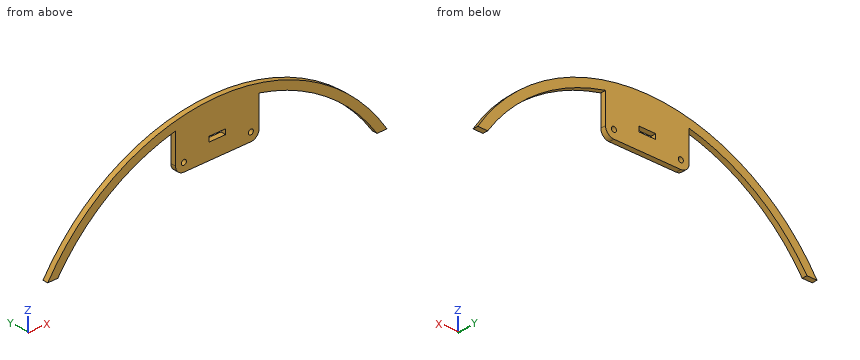
```python
from build123d import *

# Parameters (mm, degrees)
SKETCH_1_R      = 1.5
SKETCH_1_W      = 10
SKETCH_1_H      = 3
EXTRUDE_2_DEPTH = 3.125


with BuildPart() as part:
    # 草图1 → 凸台-拉伸2 (new body)
    with BuildSketch(Plane(origin=(0, 0, 0), x_dir=(1, 0, 0), z_dir=(0, 1, 0))):
        with BuildLine():
            Line((-101.350743825, 30), (-95.378054467, 30))
            ThreePointArc((-95.378054467, 30), (-64.797523096, -0.757020266), (-25, -18))
            Line((-25, -18), (-25, 0))
            ThreePointArc((-25, 0), (-23.535533906, 3.535533906), (-20, 5))
            Line((-20, 5), (20, 5))
            ThreePointArc((20, 5), (23.535533906, 3.535533906), (25, 0))
            Line((25, 0), (25, -18))
            ThreePointArc((25, -18), (64.797523096, -0.757020266), (95.378054467, 30))
            Line((95.378054467, 30), (101.350743825, 30))
            ThreePointArc((101.350743825, 30), (0, -25.750278397), (-101.350743825, 30))
        make_face()
        with Locations((-20, 0)):
            Circle(SKETCH_1_R, mode=Mode.SUBTRACT)
        with Locations((20, 0)):
            Circle(SKETCH_1_R, mode=Mode.SUBTRACT)
        with Locations((0, -6)):
            Rectangle(SKETCH_1_W, SKETCH_1_H, mode=Mode.SUBTRACT)
    extrude(amount=EXTRUDE_2_DEPTH)


solid = part.part
```
CAD build for the part. Positions are in the model's coordinates, mm. Round coordinates to 2 decimals unless told otherwise and drop trailing zeros. Order: outer loops, then holes, each group sorted by start corner. A loop starts at its lowest first (then second) coordinate and runs counter-clockwise, first axis right, second up.
Item 1: Saw through at B-B on z = 16. Write the cut outline in (x, y) (3 decimals), then the cut area to 3 significant figures.
Item 2: Saw through at C-C on z = -26. Write the cut outline in (x, y) (3 decimals), then the cut area to 3 significant figures.
Item 3: Pin check, flat tips, straight feed: pin 1 (2.5 mm diameter, centred on x = -20, z = 0, fed in from +Y); pin 2 (0.9 mm diameter, centred on x = 2.5, y = 1.5, fed in from -Z); pin 3 (1.6 mm diameter, centred on y = 1, z = 12, fed in from +X); pin 4 (1.5 mm diameter, centred on x = 27, y = 2.5, fed in from +Z). Stop position of each tip, or through.
Item 4: Saw through at D-D on x = 59. Write the cut outline in (y, z) (3 decimals), then the cut area to 3 significant figures.
Item 5: Probe line 1 along X through (y, z) = (2, 0); line 2 along Z through (x, y) = (20, 1.05); line 3 along X through (y, z) = (0.8, 7). List the from-to ranges inside material, lowest first.
Item 6: Saw through at A-A on y = 0.9. Write the cut outline in (x, z), then the cut area to 3 significant figures.
Reported:
1. outline: (-47.381, 0) - (-32.711, 0) - (-32.711, 3.125) - (-47.381, 3.125) - close; (-25, 0) - (25, 0) - (25, 3.125) - (-25, 3.125) - close; (32.711, 0) - (47.381, 0) - (47.381, 3.125) - (32.711, 3.125) - close
1. area: 248 mm2
2. outline: (-98.701, 0) - (-92.558, 0) - (-92.558, 3.125) - (-98.701, 3.125) - close; (92.558, 0) - (98.701, 0) - (98.701, 3.125) - (92.558, 3.125) - close
2. area: 38.4 mm2
3. pin 1: passes through
3. pin 2: stops at z = -5
3. pin 3: stops at x = 57.27
3. pin 4: stops at z = 22.84
4. outline: (0, 4.462) - (3.125, 4.462) - (3.125, 10.244) - (0, 10.244) - close
4. area: 18.1 mm2
5. line 1: x = -74.28 to -65.89, -25 to -21.5, -18.5 to 18.5, 21.5 to 25, 65.89 to 74.28
5. line 2: z = -5 to -1.5, 1.5 to 24.07
5. line 3: x = -64.41 to -54.53, -25 to -5, 5 to 25, 54.53 to 64.41
6. outline: (-101.35, -30) - (-95.38, -30) arc R115 cw to (-25, 18) - (-25, 0) arc R5 ccw to (-20, -5) - (20, -5) arc R5 ccw to (25, 0) - (25, 18) arc R115 cw to (95.38, -30) - (101.35, -30) arc R120 ccw to start; hole circle Ø3 at (-20, 0); hole (-5, 4.5) - (5, 4.5) - (5, 7.5) - (-5, 7.5) - close; hole circle Ø3 at (20, 0)
6. area: 2,350 mm2
